```python
from build123d import *

# Parameters (mm, degrees)
BOSS_EXTRUDE1_START = -12
SKETCH3_R           = 45
BOSS_EXTRUDE1_DEPTH = 12
SKETCH4_R           = 7
CUT_EXTRUDE1_DEPTH  = 12


with BuildPart() as part:
    # Sketch1 → Revolve2 (revolve)
    with BuildSketch(Plane(origin=(0, 0, 0), x_dir=(0, 0, -1), z_dir=(1, 0, 0)), mode=Mode.PRIVATE) as revolve2_sk:
        Polygon((-109.471153846, -8.509615385), (-59.471153846, -8.509615385), (-59.471153846, 1.490384615), (-119.471153846, 1.490384615), (-119.471153846, -18.509615385), (-109.471153846, -18.509615385), align=None)
    revolve(revolve2_sk.sketch.rotate(Axis((0, -43.509615385, 119.471153846), (0, 0, -1)), 90), axis=Axis((0, -43.509615385, 119.471153846), (0, 0, -1)))

    # Sketch3 → Boss-Extrude1 (add)
    with BuildSketch(Plane(origin=(0, 0, 59.471153846), x_dir=(-1, 0, 0), z_dir=(0, 0, -1)).offset(BOSS_EXTRUDE1_START)):
        with BuildLine():
            Line((-29.647715243, -89.834694778), (-88.936024476, -54.225378957))
            ThreePointArc((-88.936024476, -54.225378957), (-95, -43.509615385), (-88.936024476, -32.793851812))
            Line((-88.936024476, -32.793851812), (-29.647715243, 2.815464009))
            ThreePointArc((-29.647715243, 2.815464009), (0, 11.490384615), (29.647715243, 2.815464009))
            Line((29.647715243, 2.815464009), (88.936024476, -32.793851812))
            ThreePointArc((88.936024476, -32.793851812), (95, -43.509615385), (88.936024476, -54.225378958))
            Line((88.936024476, -54.225378958), (29.647715243, -89.834694778))
            ThreePointArc((29.647715243, -89.834694778), (0, -98.509615385), (-29.647715243, -89.834694778))
        make_face()
        with Locations(Location((0, -43.509615385, 0), (0, 0, 180))):
            Circle(SKETCH3_R, mode=Mode.SUBTRACT)
    extrude(amount=BOSS_EXTRUDE1_DEPTH)

    # Sketch4 → Cut-Extrude1 (cut)
    with BuildSketch(Plane(origin=(0, 0, 59.471153846), x_dir=(-1, 0, 0), z_dir=(0, 0, -1))):
        with Locations((-82.5, -43.509615385)):
            Circle(SKETCH4_R)
        with Locations((82.5, -43.509615385)):
            Circle(SKETCH4_R)
    extrude(amount=-CUT_EXTRUDE1_DEPTH, mode=Mode.SUBTRACT)


solid = part.part
```
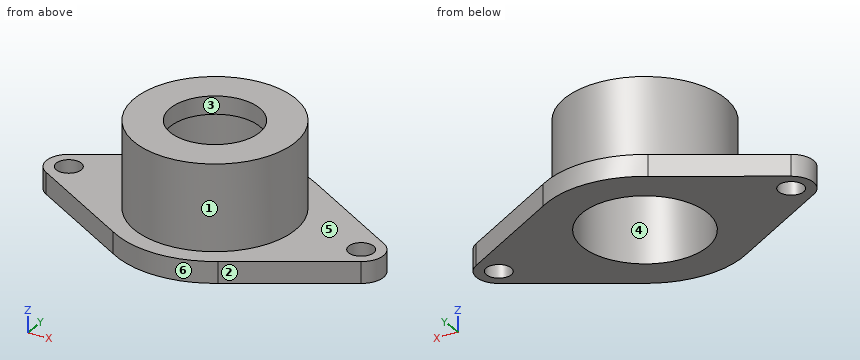
Check sheet for the modelled part. Datum: model origin and axes. Units: mm. Face numbers are marked on the shaded views. A direction names the side the tool comes from. Round coordinates to 2 decimals unless told otherwise and drop trailing zeros. Order: outer loops, then holes, each group sorted by start corner. A loop starts at its lowest first (then second) coordinate and runs counter-clockwise, first axis right, second up. Notation, with made-up numbers: M 34,14.5 L 76,14.5 A28 ccw 76,50.5 Z; hole C 22.5,40.5 d8. An arc over 180 degrees is marked long. Answer in a Markdown table with one row per item.
(1) Section check D-D on x = 27.5. Record the boundary of the cut face in (y, z).
Findings:
| item | result |
|---|---|
| outline | M -91.14,59.47 L -65.16,59.47 L -65.16,109.47 L -21.86,109.47 L -21.86,59.47 L 4.12,59.47 L 4.12,71.47 L -7.89,71.47 L -7.89,119.47 L -79.13,119.47 L -79.13,71.47 L -91.14,71.47 Z |
(2) Draft check along Y on the marked faces 1, 2, 3 and 4. Enter one of: +Y half, -Y half, draft (parallel to the pull), parting line (faces both ways), or undercut.
Findings:
| item | result |
|---|---|
| face 1 | parting line |
| face 2 | -Y half |
| face 3 | undercut |
| face 4 | undercut |
(3) Section check A-A on x = 0. Record the boundary of the cut face in (y, z), plus the area to 3 significant figures.
Findings:
| item | result |
|---|---|
| outline | M -98.51,59.47 L -78.51,59.47 L -78.51,109.47 L -68.51,109.47 L -68.51,119.47 L -88.51,119.47 L -88.51,71.47 L -98.51,71.47 Z; M -18.51,109.47 L -8.51,109.47 L -8.51,59.47 L 11.49,59.47 L 11.49,71.47 L 1.49,71.47 L 1.49,119.47 L -18.51,119.47 Z |
| area | 1,640 mm^2 |
(4) Set-up check for the marked faces 5 and 6: record each of +Z, -Z, +X, -X, +Y, -Y from which the full face is reachable in a straight line by a thin tool's end or side.
Findings:
| item | result |
|---|---|
| face 5 | +Z |
| face 6 | +Z, -Z, -Y |
(5) Section check C-C on z = 65. Record the boundary of the cut face in (x, y), plus the area to 3 significant figures.
Findings:
| item | result |
|---|---|
| outline | M -88.94,-54.23 L -29.65,-89.83 A55 ccw 29.65,-89.83 L 88.94,-54.23 A12.5 ccw 88.94,-32.79 L 29.65,2.82 A55 ccw -29.65,2.82 L -88.94,-32.79 A12.5 ccw Z; hole C -82.5,-43.51 d14; hole C 0,-43.51 d70; hole C 82.5,-43.51 d14 |
| area | 8,980 mm^2 |
(6) Gauge pin test, flat ends, axial feed: pin 1 (22.5 mm diameter, centred on x = 82.5, y = -43.51, fed in from -Z); pin 2 (3 mm diameter, centred on y = -51.5, z = 71.5, fed in from +X); pin 3 (8 mm diameter, centred on x = -34, z = 96.5, fed in from +Y); pin 4 (12 mm diameter, centred on y = -11, z = 84, fed in from +X). Record the tip position at first contact, or that the pin passes through.
Findings:
| item | result |
|---|---|
| pin 1 | stops at z = 59.47 |
| pin 2 | stops at x = 93.18 |
| pin 3 | stops at y = -9.97 |
| pin 4 | stops at x = 36.36 |
(7) Section check B-B on y = -60. Record the boundary of the cut face in (x, z), plus the area to 3 significant figures.
Findings:
| item | result |
|---|---|
| outline | M -79.32,59.47 L -30.87,59.47 L -30.87,109.47 L -18.79,109.47 L -18.79,119.47 L -41.87,119.47 L -41.87,71.47 L -79.32,71.47 Z; M 18.79,109.47 L 30.87,109.47 L 30.87,59.47 L 79.32,59.47 L 79.32,71.47 L 41.87,71.47 L 41.87,119.47 L 18.79,119.47 Z |
| area | 2,460 mm^2 |
(8) Material ranges on line 1 along Y through (x, z) = (0, 97); line 2 along Y through (x, z) = (0, 114); line 3 along X through (y, z) = (-55, 103.5), recorded low to high. Write a range as from..to.
Findings:
| item | result |
|---|---|
| line 1 | y = -88.51..-78.51, -8.51..1.49 |
| line 2 | y = -88.51..-68.51, -18.51..1.49 |
| line 3 | x = -43.51..-33.06, 33.06..43.51 |
